Can you work these out from the drawing? Everything is in mm from the part's minimum corner. A direction names the side the tool comes from. Round coordinates to 2 decimals unless told otherwise and drop trailing zeros. Write each loop counter-clockwise with the first axis right and the second up, starting at its lowest first coordinate (ties: lowest second). Pieces come first, ordered by that corner, then holes. Notation, with made-up numbers: (23.25, 25) -> (27.25, 25) arc R15 ccw to (27.25, 47) -> close; hole circle Ø7 at (57.25, 53). An arc over 180 degrees is marked (long way). Write item = value, one per line. Start each with the question number.
1) If I drill on line 1 (X direction, y = 1, z = 2); line 2 (X direction, y = 1, z = 35.5); line 3 (X direction, y = 7.5, z = 33.5), over which ranges is the centre line in solid material (lowest first)?
2) I'm going to push flat-ended pins straight in: pin 1 (2 mm diameter, centred on x = 28.5, z = 34.5, fed in from +Y); pin 2 (1 mm diameter, centred on y = 0.5, z = 20, fed in from -X); pin 3 (5 mm diameter, centred on x = 18, y = 3.5, fed in from -Z); pin 4 (2.5 mm diameter, centred on y = 7, z = 34, fed in from -X). Where does each tip first touch, or does it pass through?
3) Imagine slicing it at A-A, the plane z = 4.5. Please give me the cut outline in (x, y).
4) Thinking about a two-plate mould opening in X: for the marked faces 5, 6, 7 and 8, which applies, +X half, -X half, draft (parallel to the pull), parting line (faces both ways), or undercut?
5) Imagine slicing it at D-D, the plane z = 30.5. Please give me the cut outline in (x, y), then the cut area to 3 significant figures.
6) Imagine slicing it at C-C, the plane y = 3.5. Please give me the cut outline in (x, z), then the cut area to 3 significant figures.
7) For the marked faces 1, 2, 3 and 4, which set-ups out of +Z, -Z, +X, -X, +Y, -Y let a thin tool reach every point of the face, with its end or its side?
8) Imagine slicing it at B-B, the plane x = 27. Please give me the cut outline in (y, z), then the cut area to 3 significant figures.
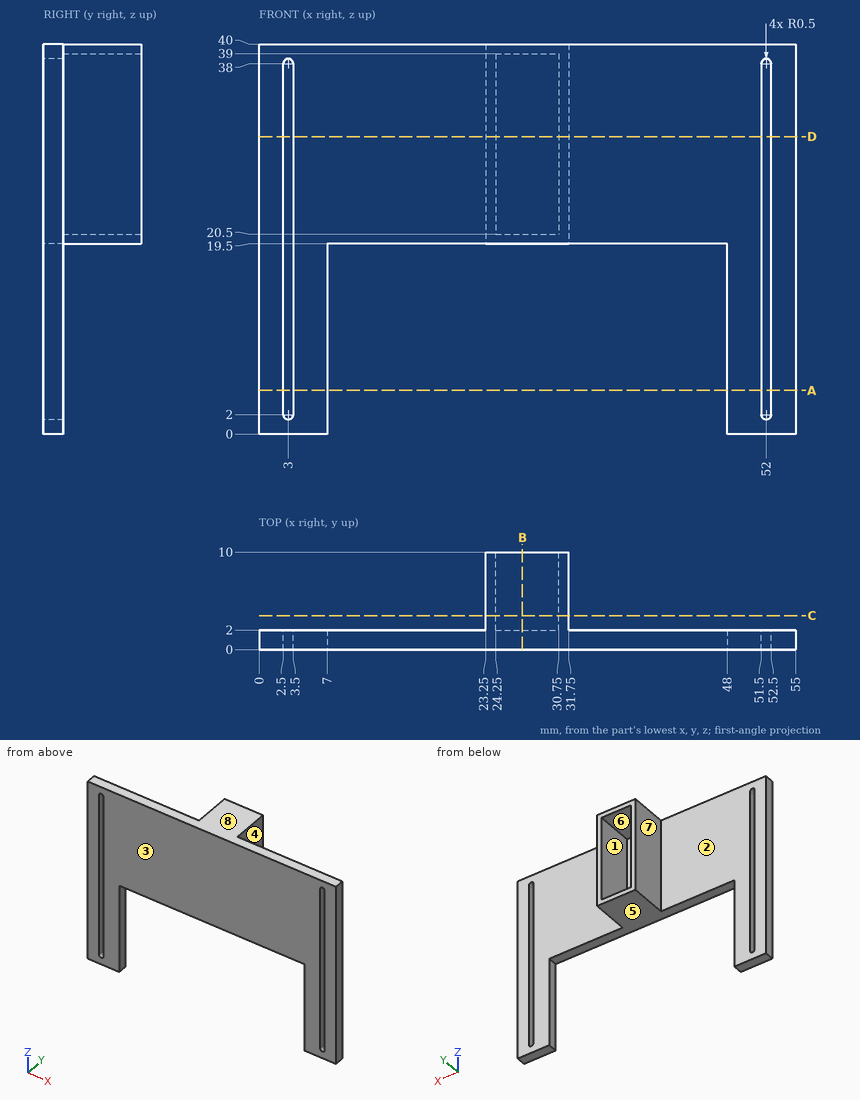
Reported:
q1.line_1 = 0 to 2.5, 3.5 to 7, 48 to 51.5, 52.5 to 55
q1.line_2 = 0 to 2.5, 3.5 to 51.5, 52.5 to 55
q1.line_3 = 23.25 to 24.25, 30.75 to 31.75
q2.pin_1 = 2
q2.pin_2 = 0
q2.pin_3 = 19.5
q2.pin_4 = 23.25
q3.outline = (0, 0) -> (2.5, 0) -> (2.5, 2) -> (0, 2) -> close; (3.5, 0) -> (7, 0) -> (7, 2) -> (3.5, 2) -> close; (48, 0) -> (51.5, 0) -> (51.5, 2) -> (48, 2) -> close; (52.5, 0) -> (55, 0) -> (55, 2) -> (52.5, 2) -> close
q4.face_5 = undercut
q4.face_6 = undercut
q4.face_7 = -X half
q4.face_8 = draft
q5.outline = (0, 0) -> (2.5, 0) -> (2.5, 2) -> (0, 2) -> close; (3.5, 0) -> (51.5, 0) -> (51.5, 2) -> (31.75, 2) -> (31.75, 10) -> (30.75, 10) -> (30.75, 2) -> (24.25, 2) -> (24.25, 10) -> (23.25, 10) -> (23.25, 2) -> (3.5, 2) -> close; (52.5, 0) -> (55, 0) -> (55, 2) -> (52.5, 2) -> close
q5.area = 122 mm²
q6.outline = (23.25, 19.5) -> (31.75, 19.5) -> (31.75, 40) -> (23.25, 40) -> close; hole (24.25, 20.5) -> (30.75, 20.5) -> (30.75, 39) -> (24.25, 39) -> close
q6.area = 54.0 mm²
q7.face_1 = +Y
q7.face_2 = +Z, -Z, -X, +Y
q7.face_3 = +Z, -Z, +X, -X, -Y
q7.face_4 = +Z, -Z, +X, +Y
q8.outline = (0, 19.5) -> (10, 19.5) -> (10, 20.5) -> (2, 20.5) -> (2, 39) -> (10, 39) -> (10, 40) -> (0, 40) -> close
q8.area = 57.0 mm²
